Answer from the drawing. Dimensions are ordinates in mm from the lowest x, y and z of the part. A direction names the side the tool comes from. Give positions to 0.01 mm unless a question says otherwise; leave off trailing zeros. Loops run counter-clockwise (first coordinate to the right, second up) from the corner with the lowest first, then second, coordinate; pieces in that order, holes last.
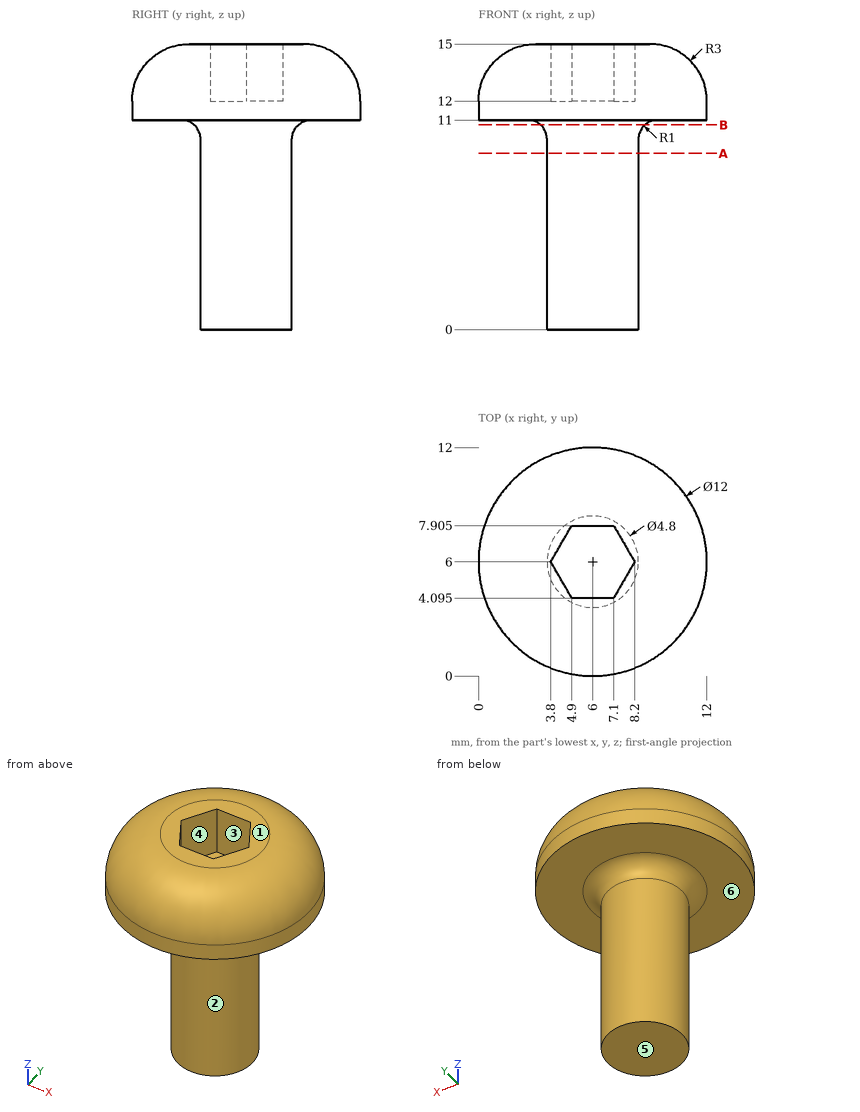
Item 1: For the marked faces 5 and 6, determine the directions among +Z, -Z, +X, -X, +Y, -Y from which every point of the face is accessible in a straight line to the end or side of a thin tool.
Item 2: Consider line 1 (Z direction, x = 5.75, y = 6); line 2 (Y direction, x = 5.25, z = 14.5) (1 decimal); line 3 (Y direction, x = 5.5, z = 12.5) (1 decimal). Determine where each line is inside the solid, lowest interval first.
Item 3: Determine the mould class of the marked faces 1, 2, 3 and 4 for opening direction Y: released by +Y, released by -Y, zero draft, split by the parting line, or undercut.
Item 4: Find section A-A, the plane z = 9.25. Write down the section's boundary in (x, y), plus the area to 3 significant figures.
Item 5: Find section B-B, the plane z = 10.75. Write down the section's boundary in (x, y), plus the area to 3 significant figures.
Item 6: Flat-ended cylindrical pins translate along their axes: pin 1 Ø6 at (y, z) = (8.5, 6.5) entering from +X; pin 2 Ø4 at (y, z) = (2, 5.5) entering from +X (1 decimal); pin 3 Ø1.1 at (x, z) = (5.5, 13.5) entering from -Y. Find the tip coordinate at first contact, or state that the pin passes through.
Ans:
1. face 5: -Z, +X, -X, +Y, -Y
1. face 6: -Z
2. line 1: z = 0 to 12
2. line 2: y = 1.4 to 4.1, 7.9 to 10.6
2. line 3: y = 0.1 to 4.1, 7.9 to 11.9
3. face 1: zero draft
3. face 2: split by the parting line
3. face 3: undercut
3. face 4: undercut
4. outline: circle Ø4.8 at (6, 6)
4. area: 18.1 mm2
5. outline: circle Ø5.48 at (6, 6)
5. area: 23.6 mm2
6. pin 1: stops at x = 8.4
6. pin 2: stops at x = 7.3
6. pin 3: stops at y = 0.17
